For this review, take the finished solid that the model builds, in its own axes (mm). A direction names the side the tool comes from. Give positions to 0.01 mm unless a question says otherwise; leave off trailing zeros. Loops run counter-clockwise (first coordinate to the right, second up) from the corner with the lowest first, then second, coordinate; pieces in that order, holes last. Notation, with made-up numbers: (-28, 57.25) -> (-16, 57.25) arc R23 cw to (-16, 70.25) -> close; hole circle Ø9 at (13, 26.5). An arc over 180 degrees is marked (long way). One line per question, with ' | ' between items. Start each with the question number.
(1) Draft analysis for pull direction Z (two halves, no side actions). For faces 1 (the flat face through (6.849, 0.74, -11.862)), 2 (the cylindrical face through (-9.246, 0.74, -3.81)), 3 (the cylindrical face through (6.727, 0.74, 16.156)), state which applies: +Z half, -Z half, draft (parallel to the pull), parting line (faces both ways), or undercut.
(2) Consider section C-C (z = -8). Write out the cut boundary in (x, y), and give its area (3 significant figures).
(3) Consider section D-D (x = 8). Write out the cut boundary in (y, z).
(4) Consider section A-A (z = -1.5). Write out the cut boundary in (x, y).
(5) Consider section B-B (x = -11). Write out the cut boundary in (y, z), and give its area (3 significant figures).
(6) Tool access review of faces 4 (the cylindrical face through (-3.81, 0.74, 9.246)), 5 (the flat face through (14, 1, 0)), 6 (the cylindrical face through (-9.912, 0.74, 1.323)): name each direction out of +Z, -Z, +X, -X, +Y, -Y from which nothing blocks a thin tool from reaching the whole face with its end or side.
(7) Insertion check: P1, Ø0.8, axis at x = -12, y = 0.5, coming from the +Z side; P2, Ø11, axis at x = 0, z = 0, coming from the +Y side. Each pin has a flat end and moves straight along its axis. Give the tip position at first contact, or say it passes through.
(8) Wall thickness on probe 1 along Z at (x, y) = (-13, 0.7); probe 2 along Z at (x, y) = (11.5, 1.2); probe 3 along X at (y, z) = (0.8, 8.5): over which ranges is each line inside the solid? List them lowest first.
Autodesk Inventor part; units mm, degrees
ref_plane "YZ Plane" through (0, 0, 0) normal (1, 0, 0) x (0, 1, 0)
ref_plane "XZ Plane" through (0, 0, 0) normal (0, 1, 0) x (-1, 0, 0)
ref_plane "XY Plane" through (0, 0, 0) normal (0, 0, 1) x (1, 0, 0)
sketch "Boceto1" plane through (0, 0, 0) normal (0, 1, 0) x (-1, 0, 0)
  line L0 (0, -10) -> (0, -17.5)
  arc A0 (0, -10) -> (2.5882, -9.6593) centre (0, 0) ccw
  line L1 (2.5882, -9.6593) -> (4.5293, -16.9037)
  line L2 (5, -8.6603) -> (8.75, -15.1554)
  arc A1 (5, -8.6603) -> (7.0711, -7.0711) centre (0, 0) ccw
  line L3 (7.0711, -7.0711) -> (12.3744, -12.3744)
  line L4 (8.6603, -5) -> (15.1554, -8.75)
  arc A2 (8.6603, -5) -> (9.6593, -2.5882) centre (0, 0) ccw
  line L5 (9.6593, -2.5882) -> (16.9037, -4.5293)
  line L6 (10, 0) -> (17.5, 0)
  arc A3 (10, 0) -> (9.6593, 2.5882) centre (0, 0) ccw
  line L7 (9.6593, 2.5882) -> (16.9037, 4.5293)
  line L8 (8.6603, 5) -> (15.1554, 8.75)
  arc A4 (8.6603, 5) -> (7.0711, 7.0711) centre (0, 0) ccw
  line L9 (7.0711, 7.0711) -> (12.3744, 12.3744)
  line L10 (5, 8.6603) -> (8.75, 15.1554)
  arc A5 (5, 8.6603) -> (2.5882, 9.6593) centre (0, 0) ccw
  line L11 (2.5882, 9.6593) -> (4.5293, 16.9037)
  line L12 (0, 10) -> (0, 17.5)
  arc A6 (0, 10) -> (-2.5882, 9.6593) centre (0, 0) ccw
  line L13 (-2.5882, 9.6593) -> (-4.5293, 16.9037)
  line L14 (-5, 8.6603) -> (-8.75, 15.1554)
  arc A7 (-5, 8.6603) -> (-7.0711, 7.0711) centre (0, 0) ccw
  line L15 (-7.0711, 7.0711) -> (-12.3744, 12.3744)
  line L16 (-8.6603, 5) -> (-15.1554, 8.75)
  arc A8 (-8.6603, 5) -> (-9.6593, 2.5882) centre (0, 0) ccw
  line L17 (-9.6593, 2.5882) -> (-16.9037, 4.5293)
  line L18 (-10, 0) -> (-17.5, 0)
  arc A9 (-10, 0) -> (-9.6593, -2.5882) centre (0, 0) ccw
  line L19 (-9.6593, -2.5882) -> (-16.9037, -4.5293)
  line L20 (-8.6603, -5) -> (-15.1554, -8.75)
  arc A10 (-8.6603, -5) -> (-7.0711, -7.0711) centre (0, 0) ccw
  line L21 (-7.0711, -7.0711) -> (-12.3744, -12.3744)
  line L22 (-5, -8.6603) -> (-8.75, -15.1554)
  arc A11 (-5, -8.6603) -> (-2.5882, -9.6593) centre (0, 0) ccw
  line L23 (-2.5882, -9.6593) -> (-4.5293, -16.9037)
  arc A12 (12.3744, 12.3744) -> (8.75, 15.1554) centre (0, 0) ccw
  arc A13 (16.9037, 4.5293) -> (15.1554, 8.75) centre (0, 0) ccw
  arc A14 (16.9037, -4.5293) -> (17.5, 0) centre (0, 0) ccw
  arc A15 (12.3744, -12.3744) -> (15.1554, -8.75) centre (0, 0) ccw
  arc A16 (4.5293, -16.9037) -> (8.75, -15.1554) centre (0, 0) ccw
  arc A17 (-4.5293, -16.9037) -> (0, -17.5) centre (0, 0) ccw
  arc A18 (-12.3744, -12.3744) -> (-8.75, -15.1554) centre (0, 0) ccw
  arc A19 (-16.9037, -4.5293) -> (-15.1554, -8.75) centre (0, 0) ccw
  arc A20 (-16.9037, 4.5293) -> (-17.5, 0) centre (0, 0) ccw
  arc A21 (-12.3744, 12.3744) -> (-15.1554, 8.75) centre (0, 0) ccw
  arc A22 (4.5293, 16.9037) -> (0, 17.5) centre (0, 0) ccw
  arc A23 (-4.5293, 16.9037) -> (-8.75, 15.1554) centre (0, 0) ccw
  line L24 (5.1962, 3) -> (7.1962, 3)
  line L25 (7.1962, 3) -> (7.1962, -3)
  line L26 (7.1962, -3) -> (5.1962, -3)
  line L27 (-5.1962, -3) -> (-7.1962, -3)
  line L28 (-7.1962, -3) -> (-7.1962, 3)
  line L29 (-7.1962, 3) -> (-5.1962, 3)
  arc A24 (5.1962, 3) -> (-5.1962, 3) centre (0, 0) ccw
  arc A25 (-5.1962, -3) -> (5.1962, -3) centre (0, 0) ccw
  dimension "d6" = 360
  dimension "d11" = 2
  dimension "d12" = 6
  dimension "d13" = 2
  dimension "d14" = 6
extrude "Extrusión1" add sketch "Boceto1" along normal blind 1.5 contours L0 A17 L23 A11 L22 A18 L21 A10 L20 A19 L19 A9 L18 A20 L17 A8 L16 A21 L15 A7 L14 A23 L13 A6 L12 A22 L11 A5 L10 A12 L9 A4 L8 A13 L7 A3 L6 A14 L5 A2 L4 A15 L3 A1 L2 A16 L1 A0 | L24 L25 L26 A25 L27 L28 L29 A24
sketch "Boceto2" plane through (0, 0, 0) normal (0, -1, 0) x (1, 0, 0)
  arc A0 (-9.6593, -2.5882) -> (-8.6603, -5) centre (0, 0) ccw
hole "Agujero1" at (0, 0, 0) direction (0, 1, 0) diameter 12 depth 8 tip angle 118
properties part number "Encoder2"
A:
1) face 1: -Z half | face 2: undercut | face 3: +Z half
2) outline: (-13.86, 0) -> (-8, 0) -> (-8, 1.5) -> (-13.86, 1.5) -> close; (-6, 0) -> (8, 0) -> (8, 1.5) -> (-6, 1.5) -> close; (13.86, 0) -> (15.56, 0) -> (15.56, 1.5) -> (13.86, 1.5) -> close | area: 32.3 mm^2
3) outline: (0, -13.86) -> (1.5, -13.86) -> (1.5, -8) -> (0, -8) -> close; (0, -6) -> (1.5, -6) -> (1.5, 8) -> (0, 8) -> close; (0, 13.86) -> (1.5, 13.86) -> (1.5, 15.56) -> (0, 15.56) -> close
4) outline: (-17.44, 0) -> (-5.81, 0) -> (-5.81, 1.5) -> (-17.44, 1.5) -> close; (5.81, 0) -> (9.89, 0) -> (9.89, 1.5) -> (5.81, 1.5) -> close
5) outline: (0, -11) -> (1.5, -11) -> (1.5, -6.35) -> (0, -6.35) -> close; (0, -2.95) -> (1.5, -2.95) -> (1.5, 0) -> (0, 0) -> close; (0, 2.95) -> (1.5, 2.95) -> (1.5, 6.35) -> (0, 6.35) -> close; (0, 11) -> (1.5, 11) -> (1.5, 13.61) -> (0, 13.61) -> close | area: 20.4 mm^2
6) face 4: +Y, -Y | face 5: +X, +Y, -Y | face 6: -X, +Y, -Y
7) P1: stops at z = 13.1 | P2: passes through
8) probe 1: z = -11.72 to -7.51, -3.48 to 0, 3.48 to 7.51 | probe 2: z = -13.19 to -11.5, -6.64 to -3.08, 0 to 3.08, 6.64 to 11.5 | probe 3: x = -15.3 to -14.72, -8.5 to 5.27, 8.5 to 14.72
